Check sheet for the drawn part. Datum: minimum x, y, z corner. Units: mm. Round coordinates to 2 decimals unless told otherwise and drop trailing zeros. Order: outer loops, then holes, each group sorted by start corner. A loop starts at its lowest first (then second) coordinate and runs counter-clockwise, first axis right, second up. Notation, with made-up numbers: M -3,86 L 26,86 A12 cw 26,90 Z; hole C -39,29 d10. An arc over 180 degrees is marked long. Use one line per item in the form item = value. Start each with the question number.
Item 1: Thickness scan on probe 1 along Z at (x, y) = (22.5, 32.5); probe 2 along Y at (x, z) = (7, 18). Record the ranges inside material, lowest first. Write a range as [from, to].
Item 2: Cross-section at B-B on z = 22.5. Enter the section's corners in (x, y).
Item 3: Go/stop test with flat-tipped pins: pin 1 Ø1 at (x, y) = (29, 39.5) entering from +Z; pin 2 Ø8 at (x, y) = (21, 11) entering from -Z; pin 3 Ø13 at (x, z) = (23.5, 29.5) entering from +Y. Record where each tip stops, or that it passes through.
Item 4: Cross-section at C-C on y = 22. Enter the section's corners in (x, z), then the cut area to 3 significant figures.
Item 5: Release check for a two-part mould opening along Z. For the marked faces 1, 2 and 3 record: +Z half, -Z half, draft (parallel to the pull), parting line (faces both ways), or undercut.
Item 6: Cross-section at A-A on x = 22.5. Enter the section's corners in (y, z), then the cut area to 3 significant figures.
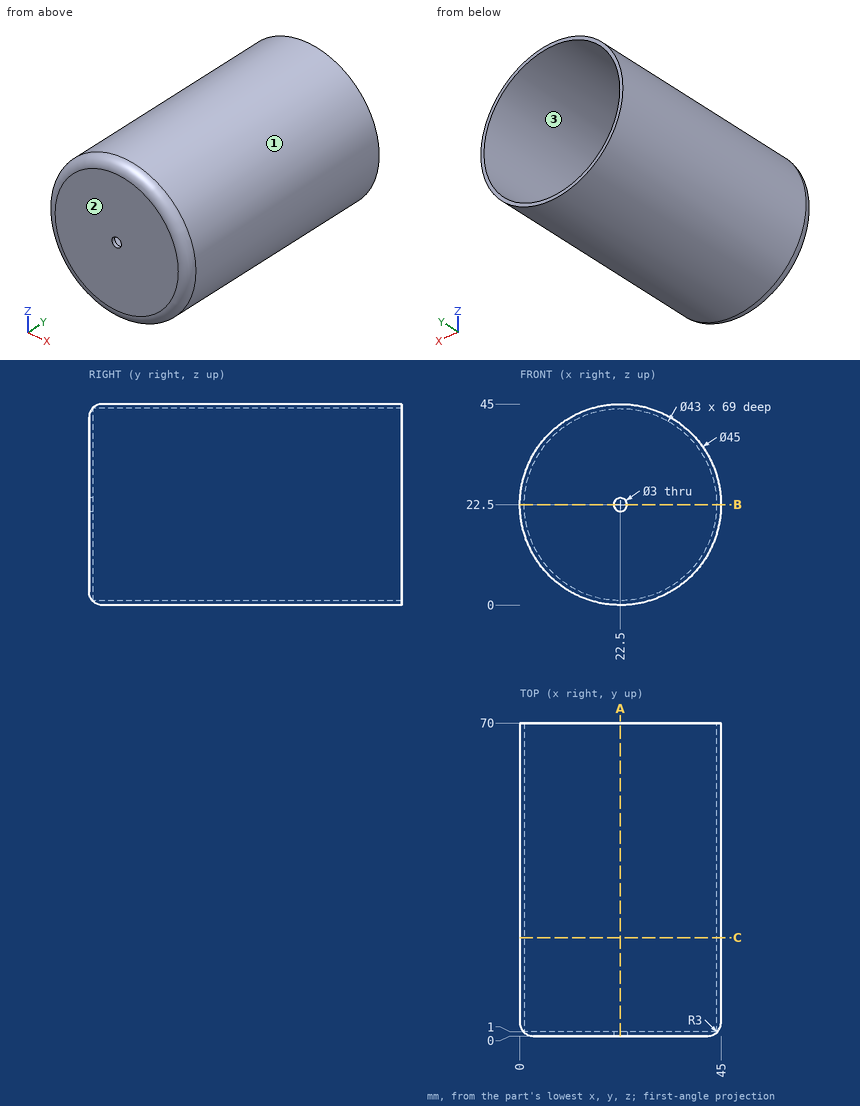
Output values:
q1.probe_1 = [0, 1], [44, 45]
q1.probe_2 = [0, 1]
q2.outline = M 0,3 A3 ccw 3,0 L 21,0 L 21,1 L 1,1 L 1,70 L 0,70 Z; M 24,0 L 42,0 A3 ccw 45,3 L 45,70 L 44,70 L 44,1 L 24,1 Z
q3.pin_1 = 44.19
q3.pin_2 = 0
q3.pin_3 = 1
q4.outline = C 22.5,22.5 d45; hole C 22.5,22.5 d43
q4.area = 138 mm2
q5.face_1 = parting line
q5.face_2 = draft
q5.face_3 = undercut
q6.outline = M 0,3 A3 ccw 3,0 L 70,0 L 70,1 L 1,1 L 1,21 L 0,21 Z; M 0,24 L 1,24 L 1,44 L 70,44 L 70,45 L 3,45 A3 ccw 0,42 Z
q6.area = 176 mm2
